The listing builds one solid part. Answer for the finished solid, in the listing's coordinates (mm). Face numbers are marked on the shaded views. Coordinates: 2 decimals unless noted, no trailing zeros. Order: outer loops, then holes, each group sorted by start corner. A loop starts at its lowest first (then second) coordinate and runs counter-clockwise, first axis right, second up. Notation, with made-up numbers: M 31,-32.75 L 87,-32.75 A28 cw 87,-14.75 Z; hole C -15,67 d10. An arc over 180 degrees is marked long. One line per item, written item: value. Start each with the question number.
Q1. The part is cut by section D-D on y = 93. Give the vertices of the cut face in (x, z).
Q2. Straight lines are drawn through the part: line 1 along X through (y, z) = (240, -0.65); line 2 along Y through (x, z) = (-101.5, 6.5); line 3 along Y through (x, z) = (-333, -0.85). For each, find the intervals that lie inside material, in ascending order. Write a range as [from, to].
Q3. The part is cut by section A-A on x = -77.5. Give the vertices of the cut face in (y, z), then the cut area to 3 significant figures.
Q4. Determine the mould class of the marked faces 1 and 2 for opening direction Y: pulls with the +Y half, pulls with the -Y half, needs draft (parallel to the pull), parting line crosses it, or undercut.
Q5. The part is cut by section C-C on x = 146. Give the vertices of the cut face in (y, z).
Q6. Each of these flat-tipped pins is pushed along its axis until it touches: pin 1 Ø1.2 at (x, z) = (-13.5, -0.5) entering from -Y; pin 2 Ø0.8 at (x, z) = (35.5, -0.5) entering from +Y. Where does it stop, or does it pass through?
Q7. The part is cut by section B-B on z = 8. Give the vertices of the cut face in (x, y), then the cut area to 3 significant figures.
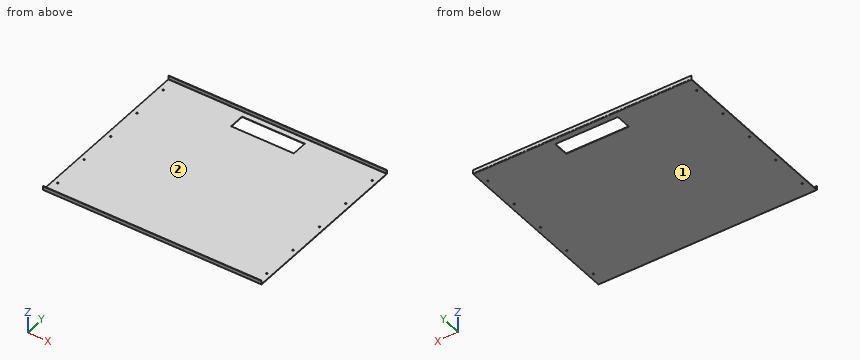
```python
from build123d import *

# Parameters (mm, degrees)
SKETCH_1_W                         = 696
SKETCH_1_H                         = 572
SM_BASE_FLANGE_1_DEPTH             = 1.5
SM_EDGE_FLANGE_1_STRIP_W           = 7.4732
SM_EDGE_FLANGE_1_STRIP_H           = 1.5
SM_EDGE_FLANGE_1_STRIP_CUT_DEPTH   = 696
SM_EDGE_FLANGE_1_STRIP_2_W         = 7.4732
SM_EDGE_FLANGE_1_STRIP_2_H         = 1.5
SM_EDGE_FLANGE_1_STRIP_CUT_2_DEPTH = 696
SM_EDGE_FLANGE_1_DEPTH             = 696
SM_EDGE_FLANGE_1_BEND_DEPTH        = 696
SKETCH_8_R                         = 2.25
CUT_EXTRUDE_1_DEPTH                = 10
PATTERN_LINEAR_1_COUNT             = 3
PATTERN_LINEAR_1_PITCH             = 120
PATTERN_LINEAR_1_COL_COUNT         = 3
PATTERN_LINEAR_1_COL_PITCH         = 120
SKETCH_9_W                         = 200
SKETCH_9_H                         = 50
CUT_EXTRUDE_2_DEPTH                = 10


# Sheet-metal steps are written as plain solids
with BuildPart() as part:
    # Sketch 1 → Базовая кромка1 (new body)
    with BuildSketch(Plane.XY):
        Rectangle(SKETCH_1_W, SKETCH_1_H)
    extrude(amount=-SM_BASE_FLANGE_1_DEPTH)

    # Ребро-кромка1 strip (across the edge) → Ребро-кромка1 strip cut (cut)
    with BuildSketch(Plane(origin=(348, 286, 0), x_dir=(0, -1, 0), z_dir=(-1, 0, 0))):
        with Locations((-1.5, -0.75)):
            Rectangle(SM_EDGE_FLANGE_1_STRIP_W, SM_EDGE_FLANGE_1_STRIP_H)
    extrude(amount=SM_EDGE_FLANGE_1_STRIP_CUT_DEPTH, mode=Mode.SUBTRACT)

    # Ребро-кромка1 strip 2 (across the edge) → Ребро-кромка1 strip cut 2 (cut)
    with BuildSketch(Plane(origin=(-348, -286, 0), x_dir=(0, 1, 0), z_dir=(1, 0, 0))):
        with Locations((-1.5, -0.75)):
            Rectangle(SM_EDGE_FLANGE_1_STRIP_2_W, SM_EDGE_FLANGE_1_STRIP_2_H)
    extrude(amount=SM_EDGE_FLANGE_1_STRIP_CUT_2_DEPTH, mode=Mode.SUBTRACT)

    # Ребро-кромка1 section (across the edge) → Ребро-кромка1 (add)
    with BuildSketch(Plane(origin=(348, 286, 0), x_dir=(0, -1, 0), z_dir=(-1, 0, 0))):
        with BuildLine():
            Line((0, 0.7366), (0, 11.5))
            Line((0, 11.5), (1.5, 11.5))
            Line((1.5, 11.5), (1.5, 0.7366))
            ThreePointArc((1.5, 0.7366), (1.715745145, 0.215745145), (2.2366, 0))
            Line((2.2366, 0), (2.2366, -1.5))
            ThreePointArc((2.2366, -1.5), (0.655084973, -0.844915027), (0, 0.7366))
        make_face()
    extrude(amount=SM_EDGE_FLANGE_1_DEPTH)

    # Ребро-кромка1 section 2 (across the edge) → Ребро-кромка1 bend (add)
    with BuildSketch(Plane(origin=(-348, -286, 0), x_dir=(0, 1, 0), z_dir=(1, 0, 0))):
        with BuildLine():
            Line((0, 0.7366), (0, 11.5))
            Line((0, 11.5), (1.5, 11.5))
            Line((1.5, 11.5), (1.5, 0.7366))
            ThreePointArc((1.5, 0.7366), (1.715745145, 0.215745145), (2.2366, 0))
            Line((2.2366, 0), (2.2366, -1.5))
            ThreePointArc((2.2366, -1.5), (0.655084973, -0.844915027), (0, 0.7366))
        make_face()
    extrude(amount=SM_EDGE_FLANGE_1_BEND_DEPTH)

    # Эскиз8 → Вырез-Вытянуть1 (cut)
    with BuildSketch(Plane.XY):
        with Locations((333, 0)):
            Circle(SKETCH_8_R)
        with Locations(Location((-333, 0, 0), (0, 0, 180))):
            Circle(SKETCH_8_R)
    cut_extrude_1 = extrude(amount=-CUT_EXTRUDE_1_DEPTH, mode=Mode.SUBTRACT)

    # Линейный массив1: Вырез-Вытянуть1 ×3
    with Locations(*[(0, -i * PATTERN_LINEAR_1_PITCH, 0) for i in range(1, PATTERN_LINEAR_1_COUNT)]):
        add(cut_extrude_1, mode=Mode.SUBTRACT)

    # Линейный массив1 col: Вырез-Вытянуть1 ×3
    with Locations(*[(0, i * PATTERN_LINEAR_1_COL_PITCH, 0) for i in range(1, PATTERN_LINEAR_1_COL_COUNT)]):
        add(cut_extrude_1, mode=Mode.SUBTRACT)

    # Эскиз9 → Вырез-Вытянуть2 (cut)
    with BuildSketch(Plane.XY):
        with Locations((0, 241)):
            Rectangle(SKETCH_9_W, SKETCH_9_H)
    extrude(amount=-CUT_EXTRUDE_2_DEPTH, mode=Mode.SUBTRACT)


solid = part.part
```
Output:
1. outline: M -348,-1.5 L 348,-1.5 L 348,0 L -348,0 Z
2. line 1: x = [-348, -335.25], [-330.75, -100], [100, 330.75], [335.25, 348]
2. line 2: y = [-286, -284.5], [284.5, 286]
2. line 3: y = [-285.34, -242.25], [-237.75, -122.25], [-117.75, -2.25], [2.25, 117.75], [122.25, 237.75], [242.25, 285.34]
3. outline: M -286,0.74 A2.24 ccw -283.76,-1.5 L 216,-1.5 L 216,0 L -283.76,0 A0.74 cw -284.5,0.74 L -284.5,11.5 L -286,11.5 Z; M 266,-1.5 L 283.76,-1.5 A2.24 ccw 286,0.74 L 286,11.5 L 284.5,11.5 L 284.5,0.74 A0.74 cw 283.76,0 L 266,0 Z
3. area: 816 mm^2
4. face 1: needs draft
4. face 2: undercut
5. outline: M -286,0.74 A2.24 ccw -283.76,-1.5 L 283.76,-1.5 A2.24 ccw 286,0.74 L 286,11.5 L 284.5,11.5 L 284.5,0.74 A0.74 cw 283.76,0 L -283.76,0 A0.74 cw -284.5,0.74 L -284.5,11.5 L -286,11.5 Z
6. pin 1: stops at y = -285.91
6. pin 2: stops at y = 285.84
7. outline: M -348,-286 L 348,-286 L 348,-284.5 L -348,-284.5 Z; M -348,284.5 L 348,284.5 L 348,286 L -348,286 Z
7. area: 2,090 mm^2
